Source: CAD feature listing. Evaluate the final solid. Frame: model axes, mm. Face numbers are marked on the shaded views. A direction names the side the tool comes from. Coordinates: 2 decimals unless noted, no trailing zeros. Loops run counter-clockwise (first coordinate to the right, second up) from the corner with the lowest first, then second, coordinate; pieces in that order, holes last.
Item 1: Section query B-B, the plane y = 37. Return the cut outline in (x, z).
Item 2: Section query D-D, the plane z = -1.5. Return the cut outline in (x, y), then the cut area to 3 significant figures.
Item 3: Pin query (flat end, axial travel): pin 1 Ø1 at (x, z) = (19.5, -3.5) entering from +Y; pin 2 Ø4 at (x, z) = (7, -16.5) entering from +Y. Return the tip coordinate at first contact, or that it passes through.
Item 4: Reachability of the marked faces 5 and 6 from +Z, -Z, +X, -X, +Y, -Y: full face, straight path, thin tool, end or side. Return the list, or none.
Item 5: Pull-direction query (X, two-part tool) for the marked faces 1, 2, 3 and 4; classes: +X half, -X half, draft (parallel to the pull), parting line (faces both ways), or undercut.
Item 6: Line query: probe 1 along X at (y, z) = (84.5, -9); probe 2 along Y at (x, z) = (-32.5, 29.5); probe 3 along Y at (x, z) = (-20.5, -10.5). Output: solid intervals per line, ascending.
Item 7: Section query A-A, the plane z = -46.5. Return the cut outline in (x, y).
Item 8: Section query C-C, the plane y = 7.5. Return the cut outline in (x, z).
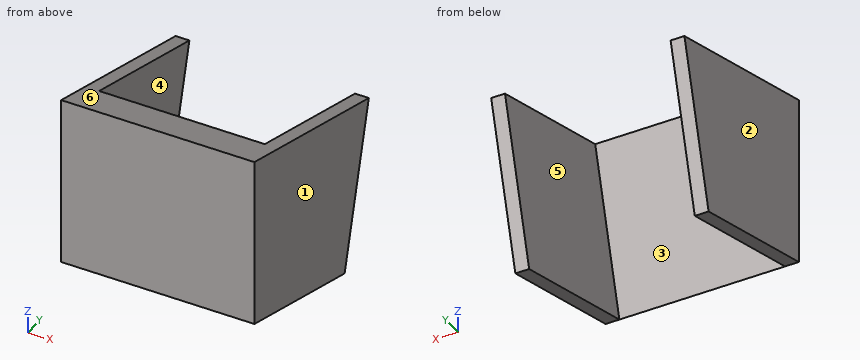
```python
from build123d import *

# Parameters (mm, degrees)
BOSS_EXTRUDE1_DEPTH = 44.45
CUT_EXTRUDE1_DEPTH  = 38.1


with BuildPart() as part:
    # Sketch1 → Boss-Extrude1 (new, symmetric)
    with BuildSketch(Plane(origin=(0, 0, 0), x_dir=(0, 0, -1), z_dir=(1, 0, 0))):
        Polygon((-39.444022474, 0), (39.444022474, 0), (59.16603371, 73.603547963), (-14.437514253, 93.3255592), align=None)
    extrude(amount=BOSS_EXTRUDE1_DEPTH, both=True)

    # Sketch2 → Cut-Extrude1 (cut, symmetric)
    with BuildSketch(Plane(origin=(0, 0, 0), x_dir=(0, 0, -1), z_dir=(1, 0, 0))):
        Polygon((-34.15952549, 19.722011237), (-14.437514253, 93.3255592), (59.16603371, 73.603547963), (39.444022474, 0), align=None)
    extrude(amount=CUT_EXTRUDE1_DEPTH, both=True, mode=Mode.SUBTRACT)


solid = part.part
```
Verdict:
1. outline: (-44.45, -49.36) - (-38.1, -49.36) - (-38.1, 29.53) - (-44.45, 29.53) - close; (38.1, -49.36) - (44.45, -49.36) - (44.45, 29.53) - (38.1, 29.53) - close
2. outline: (-44.45, 0) - (44.45, 0) - (44.45, 89.06) - (38.1, 89.06) - (38.1, 10.17) - (-38.1, 10.17) - (-38.1, 89.06) - (-44.45, 89.06) - close
2. area: 1,910 mm2
3. pin 1: stops at y = 9.77
3. pin 2: stops at y = 6.68
4. face 5: -Z, +Y
4. face 6: +Z, +X, -X, +Y
5. face 1: +X half
5. face 2: -X half
5. face 3: undercut
5. face 4: undercut
6. probe 1: x = -44.45 to -38.1, 38.1 to 44.45
6. probe 2: y = 0 to 18.47
6. probe 3: y = 0 to 7.76
7. outline: (-44.45, 26.33) - (-38.1, 26.33) - (-38.1, 77) - (-44.45, 77) - close; (38.1, 26.33) - (44.45, 26.33) - (44.45, 77) - (38.1, 77) - close
8. outline: (-44.45, -41.45) - (-38.1, -41.45) - (-38.1, -11.45) - (38.1, -11.45) - (38.1, -41.45) - (44.45, -41.45) - (44.45, 37.43) - (-44.45, 37.43) - close
